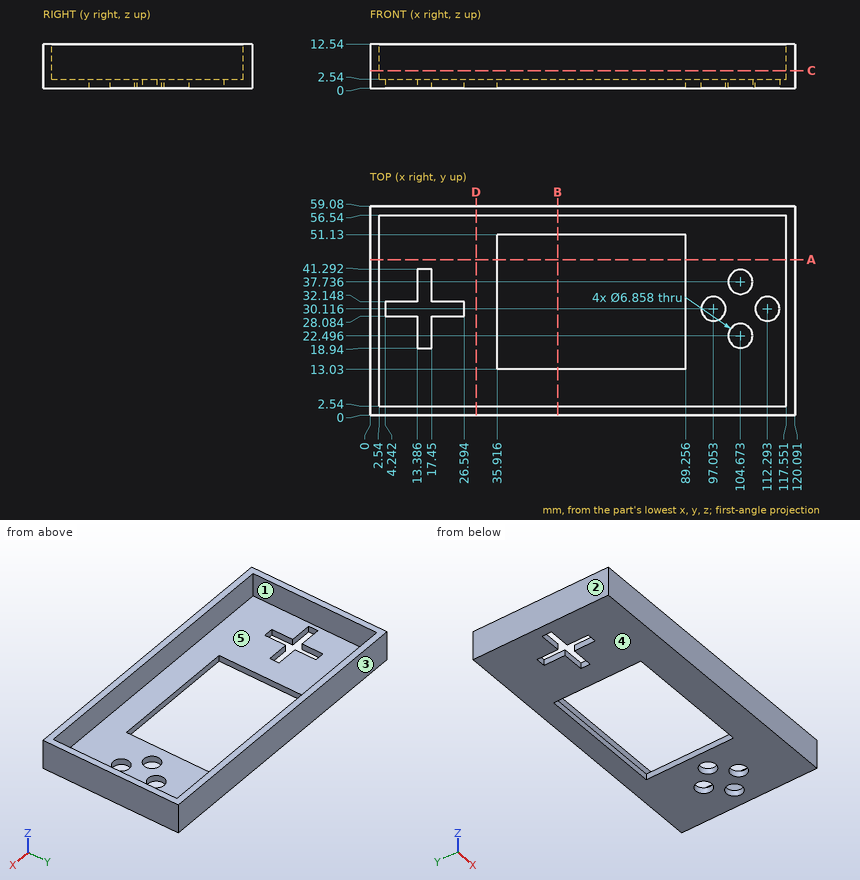
Source: three-view drawing plus pictorial views. Frame: mm from the lowest corner of the part. A direction names the side the tool comes from. Coordinates: 2 decimals unless noted, no trailing zeros. Order: outer loops, then holes, each group sorted by start corner. A loop starts at its lowest first (then second) coordinate and runs counter-clockwise, first axis right, second up.
1) Set-up query: the marked faces 4 and 5. Return all of +Z, -Z, +X, -X, +Y, -Y with unobstructed straight access to the full face (end or side cutting, diameter ignored); none if empty.
Result sheet:
face 4: -Z, +X, -X, +Y, -Y
face 5: +Z
2) Section B-B (x = 53). Return loops of the section in (y, z).
Result sheet:
outline: (0, 0) - (13.03, 0) - (13.03, 2.54) - (2.54, 2.54) - (2.54, 12.54) - (0, 12.54) - close; (51.13, 0) - (59.08, 0) - (59.08, 12.54) - (56.54, 12.54) - (56.54, 2.54) - (51.13, 2.54) - close
3) Ray query, probe 1 along X at (y, z) = (50.5, 4.25); probe 2 along Y at (x, z) = (61.5, 3.5); probe 3 along Z at (x, y) = (100.5, 32). Return the intervals inside material, ascending.
Result sheet:
probe 1: x = 0 to 2.54, 117.55 to 120.09
probe 2: y = 0 to 2.54, 56.54 to 59.08
probe 3: z = 0 to 2.54
4) First-contact query: P1, Ø6, axis at x = 104.67, y = 22.5, coming from the -Z side; P2, Ø10, axis at x = 24, y = 47, coming from the +Z side. Flat tips, straight axial feed; report the tip coordinate or a pass-through.
Result sheet:
P1: passes through
P2: stops at z = 2.54
5) Section C-C (z = 5). Return loops of the section in (x, y).
Result sheet:
outline: (0, 0) - (120.09, 0) - (120.09, 59.08) - (0, 59.08) - close; hole (2.54, 2.54) - (117.55, 2.54) - (117.55, 56.54) - (2.54, 56.54) - close
6) Section D-D (x = 30). Return loops of the section in (y, z).
Result sheet:
outline: (0, 0) - (59.08, 0) - (59.08, 12.54) - (56.54, 12.54) - (56.54, 2.54) - (2.54, 2.54) - (2.54, 12.54) - (0, 12.54) - close
7) Section A-A (y = 44). Return loops of the section in (x, z) (1 decimal).
Result sheet:
outline: (0, 0) - (35.9, 0) - (35.9, 2.5) - (2.5, 2.5) - (2.5, 12.5) - (0, 12.5) - close; (89.3, 0) - (120.1, 0) - (120.1, 12.5) - (117.6, 12.5) - (117.6, 2.5) - (89.3, 2.5) - close
8) Draft query along X for the marked faces 1, 2 and 3. Return one class per face: released by +X, released by -X, zero draft, split by the parting line, or undercut.
Result sheet:
face 1: undercut
face 2: released by -X
face 3: zero draft
